```python
from build123d import *

# Parameters (mm, degrees)
SKETCH7_W           = 50
SKETCH7_H           = 500
BOSS_EXTRUDE1_DEPTH = 4.5
FILLET1_R           = 20
SKETCH9_R           = 12.457833995
CUT_EXTRUDE2_DEPTH  = 10


with BuildPart() as part:
    # Sketch7 → Boss-Extrude1 (new, symmetric)
    with BuildSketch(Plane.XY):
        with Locations((12.3, -21.4)):
            Rectangle(SKETCH7_W, SKETCH7_H)
    extrude(amount=BOSS_EXTRUDE1_DEPTH, both=True)

    # Fillet1
    fillet1_edges = [part.edges().sort_by_distance(p)[0] for p in [
        (-12.7, 228.6, 0),
        (37.3, 228.6, 0),
        (37.3, -271.4, 0),
        (-12.7, -271.4, 0),
    ]]
    fillet(fillet1_edges, radius=FILLET1_R)

    # Sketch9 → Cut-Extrude2 (cut)
    with BuildSketch(Plane.XY.offset(4.5)):
        with Locations((12.3, -245.065350927)):
            Circle(SKETCH9_R)
    extrude(amount=-CUT_EXTRUDE2_DEPTH, mode=Mode.SUBTRACT)


solid = part.part
```
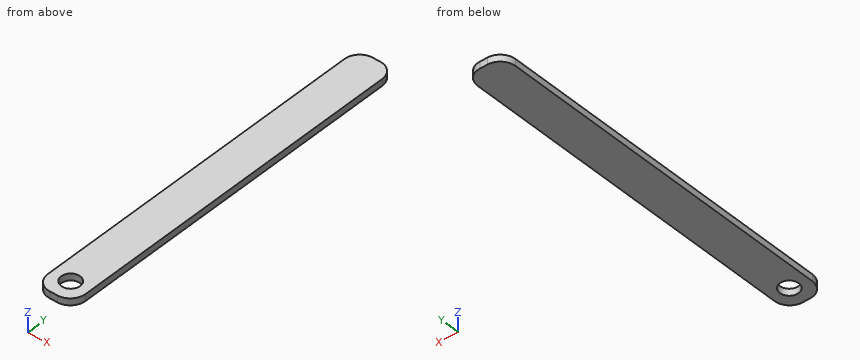
The model under review builds one solid part; all positions refer to its coordinate system, in mm. Round coordinates to 2 decimals unless told otherwise and drop trailing zeros. Write each loop counter-clockwise with the first axis right and the second up, starting at its lowest first coordinate (ties: lowest second). Pieces come first, ordered by that corner, then holes.
(1) We need section A-A on x = 12.3. Give the boundary of the cut face in (y, z), and give its area (3 significant figures).
(2) We need section B-B on z = -2. Give the boundary of the cut face in (x, y), and give its area (3 significant figures).
(3) We need section C-C on x = -6. Give the boundary of the cut face in (y, z), and give its area (3 significant figures).
(4) Insertion check: pin 1 (5 mm diameter, centred on x = 23, z = -0.5, fed in from -Y). The pin has a flat end and moves straight along its axis. Give the tip position at first contact, or say it passes through.
(5) Wall thickness on L1, parallel to Y at x = 12.3, z = 1; L2, parallel to Y at x = 14, z = -2.75; L3, parallel to Y at x = -4, z = -3.25: over which ranges is each line inside the solid? List them lowest first.
Findings below:
1. outline: (-271.4, -4.5) - (-257.52, -4.5) - (-257.52, 4.5) - (-271.4, 4.5) - close; (-232.61, -4.5) - (228.6, -4.5) - (228.6, 4.5) - (-232.61, 4.5) - close
1. area: 4,280 mm2
2. outline: (-12.7, -251.4) arc R20 ccw to (7.3, -271.4) - (17.3, -271.4) arc R20 ccw to (37.3, -251.4) - (37.3, 208.6) arc R20 ccw to (17.3, 228.6) - (7.3, 228.6) arc R20 ccw to (-12.7, 208.6) - close; hole circle Ø24.92 at (12.3, -245.07)
2. area: 24,200 mm2
3. outline: (-266.34, -4.5) - (223.54, -4.5) - (223.54, 4.5) - (-266.34, 4.5) - close
3. area: 4,410 mm2
4. pin 1: stops at y = -271.14
5. L1: y = -271.4 to -257.52, -232.61 to 228.6
5. L2: y = -271.4 to -257.41, -232.72 to 228.6
5. L3: y = -267.9 to 225.1
